Design review of the part built by this model. Coordinates are the model's own, in mm. Face numbers are marked on the shaded views. A direction names the side the tool comes from. Give positions to 0.01 mm unless a question says otherwise; leave off trailing zeros. Loops run counter-clockwise (first coordinate to the right, second up) from the corner with the lowest first, then second, coordinate; pieces in that order, holes last.
from build123d import *

# Parameters (mm, degrees)
F0_R     = 11
F0_R_2   = 5.5
F1_DEPTH = 1
F0_R_3   = 4
F2_DEPTH = 2
F3_DEPTH = 5


with BuildPart() as f1:
    # F0 (on Front) → F1 (new body)
    with BuildSketch(Plane.XZ):
        Circle(F0_R)
        Circle(F0_R_2, mode=Mode.SUBTRACT)
    extrude(amount=-F1_DEPTH)

    # F0 (on Front) → F2 (join)
    with BuildSketch(Plane.XZ):
        Circle(F0_R_2)
        Circle(F0_R_3, mode=Mode.SUBTRACT)
    extrude(amount=-F2_DEPTH)

    # F0 (on Front) → F3 (join)
    with BuildSketch(Plane.XZ):
        Circle(F0_R_3)
    extrude(amount=-F3_DEPTH)


solid = f1.part
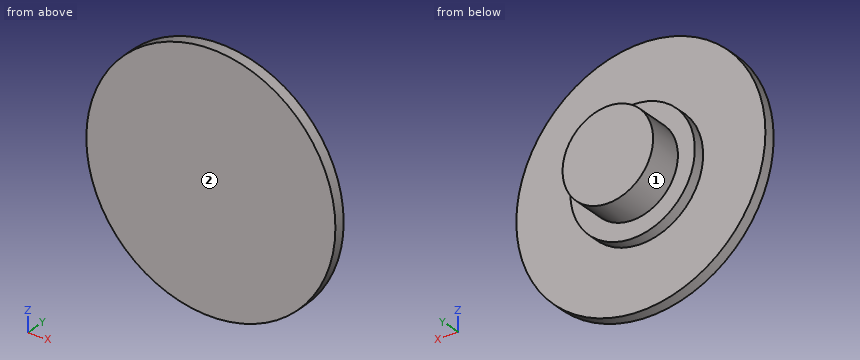
Q1. Take a section at B-B (z = 0). Give the boundary of the cut face in (x, y), plus the area to 3 significant figures.
Results:
outline: (-11, 0) - (11, 0) - (11, 1) - (5.5, 1) - (5.5, 2) - (4, 2) - (4, 5) - (-4, 5) - (-4, 2) - (-5.5, 2) - (-5.5, 1) - (-11, 1) - close
area: 57.0 mm2
Q2. Take a section at C-C (y = 2.95). Give the boundary of the cut face in (x, z), plus the area to 3 significant figures.
Results:
outline: circle Ø8 at (0, 0)
area: 50.3 mm2
Q3. Wall thickness on line 1 (Y direction, x = 0.5, z = -9.5); line 2 (X direction, y = 1.35, z = 3.5); line 3 (Z direction, x = 3, y = 1.05): over which ranges is each line inside the solid? List them lowest first.
Results:
line 1: y = 0 to 1
line 2: x = -4.24 to 4.24
line 3: z = -4.61 to 4.61
Q4. Insertion check: pin 1 (1.5 mm diameter, centred on y = 2, z = -8, fed in from +X); pin 2 (4 mm diameter, centred on x = -6.5, z = -6, fed in from +Y). Each pin has a flat end and moves straight along its axis. Give the tip position at first contact, or say it passes through.
Results:
pin 1: passes through
pin 2: stops at y = 1
Q5. Take a section at A-A (x = 0). Give the boundary of the cut face in (y, z), plus the area to 3 significant figures.
Results:
outline: (0, -11) - (1, -11) - (1, -5.5) - (2, -5.5) - (2, -4) - (5, -4) - (5, 4) - (2, 4) - (2, 5.5) - (1, 5.5) - (1, 11) - (0, 11) - close
area: 57.0 mm2
Q6. Take a section at D-D (z = -4.75). Give the boundary of the cut face in (x, y), plus the area to 3 significant figures.
Results:
outline: (-9.92, 0) - (9.92, 0) - (9.92, 1) - (2.77, 1) - (2.77, 2) - (-2.77, 2) - (-2.77, 1) - (-9.92, 1) - close
area: 25.4 mm2
Q7. Tool access review of the marked faces 1 and 2: name each direction out of +Z, -Z, +X, -X, +Y, -Y from which nothing blocks a thin tool from reaching the whole face with its end or side.
Results:
face 1: +Y
face 2: +Z, -Z, +X, -X, -Y
